from build123d import *

# Parameters (mm, degrees)
DODANIE_WYCI_GNI_CIE1_DEPTH = 6
WYTNIJ_WYCI_GNI_CIE1_REACH  = 32.34
SZKIC2_W                    = 9.7
SZKIC2_H                    = 16
SZKIC4_W                    = 10.5
SZKIC4_H                    = 23.5
WYTNIJ_WYCI_GNI_CIE3_DEPTH  = 2.5


with BuildPart() as part:
    # Szkic1 → Dodanie-wyciągnięcie1 (new body)
    with BuildSketch(Plane(origin=(0, 0, 0), x_dir=(1, 0, 0), z_dir=(0, 1, 0))):
        Polygon((-7, 10), (-7, 13.5), (7, 13.5), (7, 10), (26.5, 10), (26.5, -10), (7, -10), (7, -13.5), (-7, -13.5), (-7, -10), (-26.5, -10), (-26.5, 10), align=None)
    extrude(amount=DODANIE_WYCI_GNI_CIE1_DEPTH)

    # Szkic2 → Wytnij-wyciągnięcie1 (cut, up to next)
    with BuildSketch(Plane(origin=(0, 6, 0), x_dir=(1, 0, 0), z_dir=(0, 1, 0)), mode=Mode.PRIVATE) as wytnij_wyci_gni_cie1_sk1:
        with Locations((-19.6, 0)):
            Rectangle(SZKIC2_W, SZKIC2_H)
    wytnij_wyci_gni_cie1_tool1 = extrude(wytnij_wyci_gni_cie1_sk1.sketch, amount=-WYTNIJ_WYCI_GNI_CIE1_REACH, mode=Mode.PRIVATE) & part.part
    # Szkic2 → Wytnij-wyciągnięcie1 (cut, up to next)
    with BuildSketch(Plane(origin=(0, 6, 0), x_dir=(1, 0, 0), z_dir=(0, 1, 0)), mode=Mode.PRIVATE) as wytnij_wyci_gni_cie1_sk2:
        with Locations((19.6, 0)):
            Rectangle(SZKIC2_W, SZKIC2_H)
    wytnij_wyci_gni_cie1_tool2 = extrude(wytnij_wyci_gni_cie1_sk2.sketch, amount=-WYTNIJ_WYCI_GNI_CIE1_REACH, mode=Mode.PRIVATE) & part.part
    add(wytnij_wyci_gni_cie1_tool1.solids().sort_by_distance((-19.6, 6, 0))[0], mode=Mode.SUBTRACT)
    add(wytnij_wyci_gni_cie1_tool2.solids().sort_by_distance((19.6, 6, 0))[0], mode=Mode.SUBTRACT)

    # Szkic4 → Wytnij-wyciągnięcie3 (cut)
    with BuildSketch(Plane.XZ.offset(-6)):
        Rectangle(SZKIC4_W, SZKIC4_H)
    extrude(amount=WYTNIJ_WYCI_GNI_CIE3_DEPTH, mode=Mode.SUBTRACT)


solid = part.part
Build history of the part. All positions in model axes, mm. A direction names the side the tool comes from. Coordinates: 2 decimals unless noted, no trailing zeros. Write each loop counter-clockwise with the first axis right and the second up, starting at its lowest first coordinate (ties: lowest second). Pieces come first, ordered by that corner, then holes. Notation, with made-up numbers: (19, 15.5) -> (40, 15.5) arc R24 cw to (40, 48.5) -> close; hole circle Ø2 at (85, 89.25). An arc over 180 degrees is marked (long way). Use CSV: the item, a comma, the result in double quotes. Start each with the question number.
Q1. Flat gauge pins, fed straight in: pin 1 Ø3 at (x, y) = (-13.5, 4) entering from +Z; pin 2 Ø3 at (y, z) = (3, 12) entering from -X; pin 3 Ø8 at (x, z) = (-4, 0) entering from -Y. Where does each tip first touch, or does it go through?
Q2. 3-axis set-ups, long thin cutter, end or side, ignore diameter. For faces 1 (the flat face through (-5.25, 5, 0)), 2 (the flat face through (-20, 3, 8)), 3 (the flat face through (-17, 3, -10)): which of +Z, -Z, +X, -X, +Y, -Y reach the whole face in a straight line?
Q3. Cut at B-B, the plane z = -6.25. List the corners of the cut face in (x, y).
Q4. Pull direction X, two halves, no side cores. Call faces 4 (the flat face through (0, 3, -13.5)), 5 (the flat face through (7, 3, -12)), 6 (the flat face through (-26.5, 3, 0)), 7 (the flat face through (20, 3, 8)): released by +X, released by -X, zero draft, split by the parting line, or undercut.
Q5. Drill centre lines: probe 1 along X at (y, z) = (2.9, 4.75); probe 2 along X at (y, z) = (4.25, 0.5); probe 3 along Z at (x, y) = (21.5, 3.8). Where is each one in solid material? Low to high.
Q6. Cut at C-C, the plane y = 4. List the corners of the cut face in (x, z), then the cut area to 3 significant figures.
Q7. Cut at A-A, the plane x = 18. List the corners of the cut face in (y, z).
Checked values:
1,pin 1,"stops at z = 10"
1,pin 2,"stops at x = -7"
1,pin 3,"stops at y = 0"
2,face 1,"+Y"
2,face 2,"+Y, -Y"
2,face 3,"-Z, -X, +Y, -Y"
3,outline,"(-26.5, 0) -> (-24.45, 0) -> (-24.45, 6) -> (-26.5, 6) -> close; (-14.75, 0) -> (14.75, 0) -> (14.75, 6) -> (5.25, 6) -> (5.25, 3.5) -> (-5.25, 3.5) -> (-5.25, 6) -> (-14.75, 6) -> close; (24.45, 0) -> (26.5, 0) -> (26.5, 6) -> (24.45, 6) -> close"
4,face 4,"zero draft"
4,face 5,"released by +X"
4,face 6,"released by -X"
4,face 7,"undercut"
5,probe 1,"x = -26.5 to -24.45, -14.75 to 14.75, 24.45 to 26.5"
5,probe 2,"x = -26.5 to -24.45, -14.75 to -5.25, 5.25 to 14.75, 24.45 to 26.5"
5,probe 3,"z = -10 to -8, 8 to 10"
6,outline,"(-26.5, -10) -> (-7, -10) -> (-7, -13.5) -> (7, -13.5) -> (7, -10) -> (26.5, -10) -> (26.5, 10) -> (7, 10) -> (7, 13.5) -> (-7, 13.5) -> (-7, 10) -> (-26.5, 10) -> close; hole (-24.45, -8) -> (-14.75, -8) -> (-14.75, 8) -> (-24.45, 8) -> close; hole (-5.25, -11.75) -> (5.25, -11.75) -> (5.25, 11.75) -> (-5.25, 11.75) -> close; hole (14.75, -8) -> (24.45, -8) -> (24.45, 8) -> (14.75, 8) -> close"
6,area,"601 mm²"
7,outline,"(0, -10) -> (6, -10) -> (6, -8) -> (0, -8) -> close; (0, 8) -> (6, 8) -> (6, 10) -> (0, 10) -> close"
